Build history of the part. All positions in model axes, mm. Face numbers are marked on the shaded views. A direction names the side the tool comes from. Coordinates: 2 decimals unless noted, no trailing zeros. Loops run counter-clockwise (first coordinate to the right, second up) from the corner with the lowest first, then second, coordinate; pieces in that order, holes last.
Item 1: Cut at C-C (z = 13). Count the separate pieces of the cut face and the enclosed holes in it, and give its area (3 significant figures).
Item 2: Mould opens along Y. For the marked faces 1, 2, 3 and 4 say: released by +Y, released by -Y, zero draft, split by the parting line, or undercut.
Item 3: Flat gauge pins, fed straight in: pin 1 (4 mm diameter, centred on y = 21, z = 8, fed in from +X); pin 2 (1.6 mm diameter, centred on x = 37, z = 3, fed in from +Y); pin 3 (1 mm diameter, centred on x = 15.5, z = 2.5, fed in from +Y); pin 4 (7 mm diameter, centred on y = 10, z = 10, fed in from +X). Where does each tip first touch, or does it go through?
Item 4: Cut at D-D (y = 48). List the corners of the cut face in (x, z).
Item 5: Cut at A-A (x = 8). List the corners of the cut face in (y, z), and give its area (3 significant figures).
Item 6: 3-axis set-ups, long thin cutter, end or side, ignore diameter. For the marked faces 5 and 6: which of +Z, -Z, +X, -X, +Y, -Y reach the whole face in a straight line?
Item 7: Drill centre lines: line 1 along Z through (x, y) = (16, 54.65); line 2 along Z through (x, y) = (39, 45); line 3 along X through (y, z) = (44, 10). Where is each one in solid material? Low to high.
Item 8: Cut at B-B (y = 55). List the corners of the cut face in (x, z).
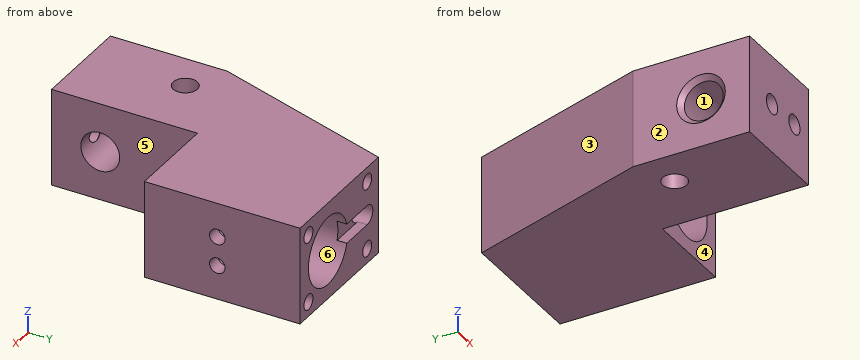
Autodesk Inventor part; units mm, degrees
ref_plane "Work Plane1" through (12, 32, 0) normal (0, 1, 0) x (1, 0, 0)
ref_plane "YZ Plane" through (0, 0, 0) normal (1, 0, 0) x (0, 1, 0)
ref_plane "XZ Plane" through (0, 0, 0) normal (0, 1, 0) x (-1, 0, 0)
sketch "Sketch1" plane through (0, 0, 0) normal (0, 0, 1) x (1, 0, 0)
  line L0 (0, 0) -> (0, 24)
  line L1 (0, 0) -> (21, 0)
  line L2 (21, 0) -> (21, 30)
  line L3 (21, 30) -> (40, 30)
  line L4 (40, 30) -> (40, 62)
  line L5 (40, 62) -> (12, 62)
  line L6 (12, 62) -> (0, 24)
  dimension "d0" = 24
  dimension "d1" = 21
  dimension "d2" = 30
  dimension "d3" = 19
  dimension "d4" = 32
  dimension "d5" = 28
extrude "Extrusion1" add sketch "Sketch1" along normal blind 20
sketch "Sketch2" plane through (12, 62, 0) normal (0, 1, 0) x (1, 0, 0)
  line L0 (28, 0) -> (28, -20)
  line L1 (28, -10) -> (18, -10)
  line L2 (28, 0) -> (28, -20)
  line L3 (28, -20) -> (0, -20)
  line L4 (0, -20) -> (0, 0)
  line L5 (0, 0) -> (28, 0)
  line L6 (28, 0) -> (28, -20)
  line L7 (28, -20) -> (0, -20)
  line L8 (0, -20) -> (0, 0)
  line L9 (0, 0) -> (28, 0)
  circle A0 centre (24, -17) radius 1.5
  circle A1 centre (24, -3) radius 1.5
  circle A2 centre (4, -3) radius 1.5
  circle A3 centre (4, -17) radius 1.5
  point P0 (-12, 0)
  point P1 (14, -10)
  dimension "d8" = 10
  dimension "d18" = 3
  dimension "d19" = 3
  dimension "d20" = 3
hole "Hole1" at (30, 62, 10) direction (0, -1, 0) diameter 14 end through all
sketch "Sketch3" plane through (12, 62, 0) normal (0, 1, 0) x (1, 0, 0)
  line L0 (28, 0) -> (28, -20)
  line L1 (28, -20) -> (25, -20)
  line L2 (28, -20) -> (0, -20)
  line L3 (25, -20) -> (25, 0)
  line L4 (28, 0) -> (0, 0)
  line L5 (25, 0) -> (4, 0)
  line L6 (4, 0) -> (4, -20)
  line L7 (4, -20) -> (25, -20)
  line L8 (4, -10) -> (4, -17)
  line L9 (4, -17) -> (25, -17)
  line L10 (25, -17) -> (25, -3)
  line L11 (25, -3) -> (4, -3)
  point P0 (-12, 0)
  dimension "d21" = 3
  dimension "d22" = 21
  dimension "d23" = 7
hole "Hole2" at (37, 62, 17) at (37, 62, 3) at (16, 62, 3) at (16, 62, 17) direction (0, -1, 0) diameter 3.2 depth 6
sketch "Sketch4" plane through (12, 62, 0) normal (0, 1, 0) x (1, 0, 0)
  point P0 (-12, 0)
sketch "Sketch5" plane through (12, 62, 0) normal (0, 1, 0) x (1, 0, 0)
  circle A0 centre (18, -10) radius 7
  circle A1 centre (4, -10) radius 2
  line L0 (4, -12) -> (11.2918, -12)
  line L1 (4, -8) -> (11.2918, -8)
  point P0 (-12, 0)
  dimension "d32" = 4
extrude "Extrusion2" cut sketch "Sketch5" against normal blind 2 contours A0 L0 A1 L1
sketch "Sketch6" plane through (12, 62, 0) normal (0, 1, 0) x (1, 0, 0)
  arc A0 (4, -12) -> (4, -8) centre (4, -10) ccw
  circle A1 centre (4, -10) radius 2
  point P0 (-12, 0)
extrude "Extrusion3" cut sketch "Sketch6" against normal blind 30
sketch "Sketch7" plane through (0, 0, 0) normal (-1, 0, 0) x (0, 0, 1)
  line L0 (0, 0) -> (20, 0)
  line L1 (10, 0) -> (10, 10)
  dimension "d37" = 10
hole "Hole3" at (0, 10, 10) direction (1, 0, 0) diameter 8 end through all countersink diameter 10 countersink angle 90
sketch "Sketch8" plane through (0, 0, 20) normal (0, 0, 1) x (1, 0, 0)
  line L0 (0, 24) -> (0, 0)
  line L1 (0, 0) -> (0, 20)
  line L2 (0, 20) -> (8, 20)
  dimension "d45" = 20
  dimension "d46" = 8
hole "Hole4" at (8, 20, 20) direction (0, 0, -1) diameter 5 end through all
ref_plane "Work Plane1" through (12, 32, 0) normal (0, 1, 0) x (1, 0, 0)
sketch "Sketch9" plane through (12, 32, 0) normal (0, 1, 0) x (1, 0, 0)
  arc A0 (4, -12) -> (4, -8) centre (4, -10) ccw
  circle A1 centre (4, -10) radius 1.25
  point P0 (-12, 0)
  dimension "d55" = 2.5
hole "Hole5" at (16, 32, 10) direction (0, -1, 0) diameter 2.5 depth 18 tip angle 118
hole "Hole6" at (16, 62, 17) at (37, 62, 17) at (37, 62, 3) at (16, 62, 3) direction (0, -1, 0) diameter 3 depth 9 tip angle 118
hole "Hole7" at (16, 62, 17) at (37, 62, 17) at (37, 62, 3) at (16, 62, 3) direction (0, -1, 0) diameter 3 depth 9 tip angle 118
sketch "Sketch10" plane through (0, 0, 0) normal (0, -1, 0) x (1, 0, 0)
  line L0 (0, 5) -> (0, 15)
  line L1 (0, 10) -> (8, 10)
  arc A0 (16, 12) -> (16, 8) centre (16, 10) ccw
  line L2 (8, 10) -> (16, 10)
  point P0 (0, 0)
  dimension "d77" = 8
  dimension "d78" = 8
hole "Hole8" at (8, 0, 10) at (16, 0, 10) direction (0, 1, 0) diameter 4 depth 6 tip angle 118
sketch "Sketch11" plane through (40, 30, 0) normal (1, 0, 0) x (0, 0, -1)
  line L0 (-12, 32) -> (-8, 32)
  line L1 (-10, 32) -> (-10, 15)
  line L2 (-10, 15) -> (-13, 15)
  line L3 (-13, 15) -> (-7, 15)
  point P0 (0, -30)
  dimension "d86" = 17
  dimension "d87" = 3
  dimension "d88" = 6
hole "Hole9" at (40, 45, 13) at (40, 45, 7) direction (-1, 0, 0) diameter 3.2 depth 3 tip angle 118
properties part number "MOTORBLOCK PART 3" material "Steel ASTM A36"
Filled sheet:
1. separate pieces: 4
1. enclosed holes: 1
1. area: 1,130 mm2
2. face 1: undercut
2. face 2: zero draft
2. face 3: released by +Y
2. face 4: released by -Y
3. pin 1: stops at x = 21
3. pin 2: stops at y = 52.58
3. pin 3: stops at y = 52.82
3. pin 4: passes through
4. outline: (7.58, 0) - (40, 0) - (40, 20) - (7.58, 20) - close; hole circle Ø4 at (16, 10); hole circle Ø14 at (30, 10)
5. outline: (0, 0) - (17.5, 0) - (17.5, 20) - (0, 20) - (0, 12) - (6, 12) - (6.3, 11.51) arc R4 cw (long way) to (6.3, 8.49) - (6, 8) - (0, 8) - close; (22.5, 0) - (49.33, 0) - (49.33, 20) - (22.5, 20) - close
5. area: 812 mm2
6. face 5: +Z, -Z, +X, -Y
6. face 6: +Y, -Y
7. line 1: z = 0 to 1.5, 4.5 to 8, 12 to 15.5, 18.5 to 20
7. line 2: z = 0 to 5.4, 8.6 to 11.4, 14.6 to 20
7. line 3: x = 6.32 to 14, 18 to 23, 37 to 40
8. outline: (9.79, 0) - (40, 0) - (40, 20) - (9.79, 20) - close; hole circle Ø4 at (16, 10); hole circle Ø3 at (16, 3); hole circle Ø3 at (16, 17); hole circle Ø14 at (30, 10); hole circle Ø3 at (37, 3); hole circle Ø3 at (37, 17)
